from build123d import *

# Parameters (mm, degrees)
BOSS_EXTRUDE1_DEPTH = 12.7
BOSS_EXTRUDE2_DEPTH = 15.24
BOSS_EXTRUDE3_DEPTH = 3.175
FILLET1_R           = 5.08
FILLET3_R           = 2.54
CHAMFER2_SIZE       = 1.27


with BuildPart() as part:
    # Sketch1 → Boss-Extrude1 (new body)
    with BuildSketch(Plane.XY):
        Polygon((74.93, -72.263), (74.93, -78.613), (-81.28, -78.613), (-81.28, 78.613), (74.93, 78.613), (74.93, 72.263), (-74.93, 72.263), (-74.93, -72.263), align=None)
    extrude(amount=BOSS_EXTRUDE1_DEPTH)

    # Sketch2 → Boss-Extrude2 (add)
    with BuildSketch(Plane(origin=(0, 0, 0), x_dir=(-1, 0, 0), z_dir=(0, 0, -1))):
        Polygon((-74.93, -65.913), (-74.93, -78.613), (81.28, -78.613), (81.28, 78.613), (-74.93, 78.613), (-74.93, 65.913), (68.58, 65.913), (68.58, -65.913), align=None)
    extrude(amount=BOSS_EXTRUDE2_DEPTH)

    # Sketch3 → Boss-Extrude3 (add)
    with BuildSketch(Plane(origin=(0, 0, -15.24), x_dir=(-1, 0, 0), z_dir=(0, 0, -1))):
        Polygon((-74.93, -53.213), (-74.93, -78.613), (81.28, -78.613), (81.28, 78.613), (-74.93, 78.613), (-74.93, 53.213), (55.88, 53.213), (55.88, -53.213), align=None)
    extrude(amount=BOSS_EXTRUDE3_DEPTH)

    # Fillet1
    fillet1_edges = [part.edges().sort_by_distance(p)[0] for p in [
        (-81.28, -78.613, -2.8575),
        (-81.28, 78.613, -2.8575),
    ]]
    fillet(fillet1_edges, radius=FILLET1_R)

    # Fillet3
    fillet3_edges = [part.edges().sort_by_distance(p)[0] for p in [
        (-55.88, 53.213, -16.8275),
        (-55.88, -53.213, -16.8275),
    ]]
    fillet(fillet3_edges, radius=FILLET3_R)

    # Chamfer2
    chamfer2_edges = [part.edges().sort_by_distance(p)[0] for p in [
        (0, -72.263, 12.7),
        (-74.93, 0, 12.7),
        (0, 72.263, 12.7),
    ]]
    chamfer(chamfer2_edges, length=CHAMFER2_SIZE)


solid = part.part
Source: CAD feature listing. Evaluate the final solid. Frame: model axes, mm. A direction names the side the tool comes from. Round coordinates to 2 decimals unless told otherwise and drop trailing zeros. Loops run counter-clockwise (first coordinate to the right, second up) from the corner with the lowest first, then second, coordinate; pieces in that order, holes last. Notation, with made-up numbers: (23.25, 21.25) -> (30.25, 21.25) arc R19 ccw to (30.25, 29.25) -> close; hole circle Ø1 at (-23.5, -12). An arc over 180 degrees is marked (long way). Answer as a JSON object with one key per item and string values. Group by question number.
Q1. Section query A-A (x = 3). Output: boundary loops of the cut face in (y, z) (3 decimals), plus the area to 3 significant figures.
Q2. Contact query for flat-ended pins moving along their axis: P1, Ø5.5, axis at y = -18, z = 7, coming from the +X side; P2, Ø12, axis at y = -3, z = -11, coming from the +X side; P3, Ø1.5, axis at y = 3.5, z = -5, coming from the +X side; P4, Ø4, axis at x = 51, y = -50.5, coming from the -Z side. Output: stop coordinate, or through.
Q3. Access query for faces 5 (the flat face through (1, 72.263, 6)), 6 (the flat face through (74.93, 72, -6)). Directions: +Z, -Z, +X, -X, +Y, -Y. A direction counts if a zero-diameter tool reaches every point of the face in a straight line with its end or side. Return the directions, or none.
Q4. Section query D-D (z = -9.5). Output: boundary loops of the cut face in (x, y), plus the area to 3 significant figures.
Q5. Mould query, pull axis Y, two halves, no side actions, for faces 1 (the flat face through (-72, 0, 0)), 2 (the flat face through (0, -78.613, -3)), 3 (the flat face through (-2, 78.613, -3)), 4 (the flat face through (-60, 5, -15.24)). Classes: pulls with the +Y half, pulls with the -Y half, needs draft (parallel to the pull), parting line crosses it, or undercut.
Q6. Section query B-B (z = 2.5). Output: boundary loops of the cut face in (x, y).
Q7. Section query C-C (y = 33). Output: boundary loops of the cut face in (x, z) (3 decimals), plus the area to 3 significant figures.
Q8. Ray query, line 1 (Y direction, x = -26, z = 7); line 2 (Y direction, x = -21, z = -15); line 3 (X direction, y = -5.5, z = -6). Return the intervals inside material, ascending. Write a range as from..to.
Completed:
{
 "1": {"outline": "(-78.613, -18.415) -> (-53.213, -18.415) -> (-53.213, -15.24) -> (-65.913, -15.24) -> (-65.913, 0) -> (-72.263, 0) -> (-72.263, 11.43) -> (-73.533, 12.7) -> (-78.613, 12.7) -> close; (53.213, -18.415) -> (78.613, -18.415) -> (78.613, 12.7) -> (73.533, 12.7) -> (72.263, 11.43) -> (72.263, 0) -> (65.913, 0) -> (65.913, -15.24) -> (53.213, -15.24) -> close", "area": "708 mm²"},
 "2": {"P1": "x = -74.93", "P2": "x = -55.88", "P3": "x = -68.58", "P4": "through"},
 "3": {"face 5": "+Z, +X", "face 6": "+Z, -Z, +X, +Y, -Y"},
 "4": {"outline": "(-81.28, -73.53) arc R5.08 ccw to (-76.2, -78.61) -> (74.93, -78.61) -> (74.93, -65.91) -> (-68.58, -65.91) -> (-68.58, 65.91) -> (74.93, 65.91) -> (74.93, 78.61) -> (-76.2, 78.61) arc R5.08 ccw to (-81.28, 73.53) -> close", "area": "5,630 mm²"},
 "5": {"face 1": "undercut", "face 2": "pulls with the -Y half", "face 3": "pulls with the +Y half", "face 4": "undercut"},
 "6": {"outline": "(-81.28, -73.53) arc R5.08 ccw to (-76.2, -78.61) -> (74.93, -78.61) -> (74.93, -72.26) -> (-74.93, -72.26) -> (-74.93, 72.26) -> (74.93, 72.26) -> (74.93, 78.61) -> (-76.2, 78.61) arc R5.08 ccw to (-81.28, 73.53) -> close"},
 "7": {"outline": "(-81.28, -18.415) -> (-55.88, -18.415) -> (-55.88, -15.24) -> (-68.58, -15.24) -> (-68.58, 0) -> (-74.93, 0) -> (-74.93, 11.43) -> (-76.2, 12.7) -> (-81.28, 12.7) -> close", "area": "354 mm²"},
 "8": {"line 1": "-78.61..-72.26, 72.26..78.61", "line 2": "-78.61..-65.91, 65.91..78.61", "line 3": "-81.28..-68.58"}
}
